Source: three-view drawing plus pictorial views. Frame: mm from the lowest corner of the part. A direction names the side the tool comes from. Give positions to 0.01 mm unless a question says otherwise; leave off trailing zeros. Order: outer loops, then holes, each group sorted by start corner. A loop starts at its lowest first (then second) coordinate and runs counter-clockwise, first axis right, second up. Notation, with made-up numbers: (-6.5, 72.5) - (37.5, 72.5) arc R17 ccw to (37.5, 87.5) - close; hole circle Ø6 at (-21, 29.5). An arc over 180 degrees is marked (long way). Use CSV: the item, a comma, the result in double quotes.
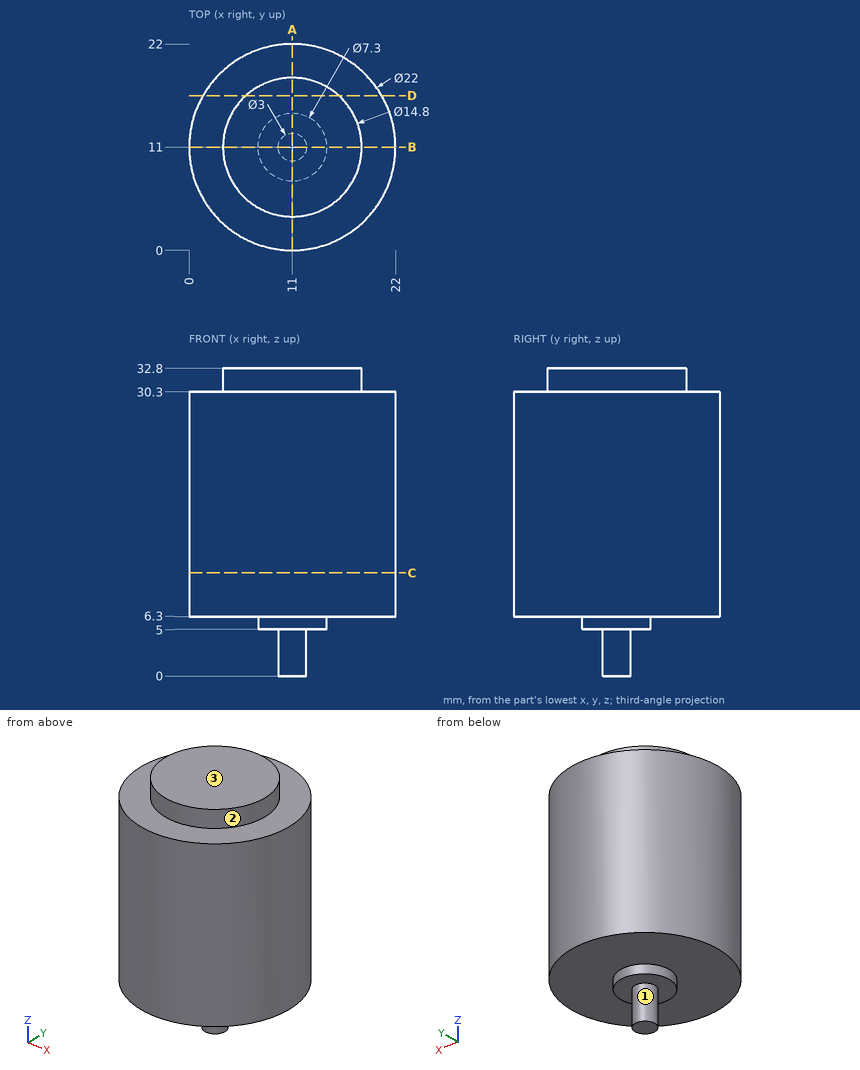
Item 1: Section A-A on x = 11. Return the cut outline in (y, z).
Filled in:
outline,"(0, 6.3) - (7.35, 6.3) - (7.35, 5) - (9.5, 5) - (9.5, 0) - (12.5, 0) - (12.5, 5) - (14.65, 5) - (14.65, 6.3) - (22, 6.3) - (22, 30.3) - (18.4, 30.3) - (18.4, 32.8) - (3.6, 32.8) - (3.6, 30.3) - (0, 30.3) - close"
Item 2: Material intervals for line 1 (Z direction, x = 17.5, y = 9.25); line 2 (Z direction, x = 14.75, y = 1.5); line 3 (Y direction, x = 20.5, z = 13.5), sorted ascending. Write a range as from..to.
Filled in:
line 1,"z = 6.3..32.8"
line 2,"z = 6.3..30.3"
line 3,"y = 5.45..16.55"
Item 3: Section C-C on z = 11. Return the cut outline in (x, y).
Filled in:
outline,"circle Ø22 at (11, 11)"
Item 4: First-contact query: pin 1 (3 mm diameter, centred on y = 6.5, z = 20.5, fed in from -X); pin 2 (10 mm diameter, centred on x = 4, z = 12, fed in from -Y); pin 3 (1 mm diameter, centred on x = 7.5, z = 26, fed in from +Y). Flat tips, straight axial feed; report the tip coordinate or a pass-through.
Filled in:
pin 1,"stops at x = 0.42"
pin 2,"stops at y = 0.18"
pin 3,"stops at y = 21.58"
Item 5: Section D-D on y = 16.5. Return the cut outline in (x, z), then the cut area to 3 significant figures.
Filled in:
outline,"(1.47, 6.3) - (20.53, 6.3) - (20.53, 30.3) - (15.95, 30.3) - (15.95, 32.8) - (6.05, 32.8) - (6.05, 30.3) - (1.47, 30.3) - close"
area,"482 mm2"
Item 6: Set-up query: the marked faces 1, 2 and 3. Return all of +Z, -Z, +X, -X, +Y, -Y with unobstructed straight access to the full face (end or side cutting, diameter ignored); none if empty.
Filled in:
face 1,"-Z"
face 2,"+Z"
face 3,"+Z, +X, -X, +Y, -Y"
